Drawing for the job (mm, zero at the part's lowest x, y, z). A direction names the side the tool comes from. Round coordinates to 2 decimals unless told otherwise and drop trailing zeros. Write each loop counter-clockwise with the first axis right and the second up, starting at its lowest first coordinate (ties: lowest second). Pieces come first, ordered by that corner, then holes. Notation, with made-up numbers: (76, -28) - (108, -28) arc R18 cw to (108, -2) - close; hole circle Ø6 at (40.25, 53.25). An arc over 180 degrees is marked (long way). Answer in a Markdown table with one row per item.
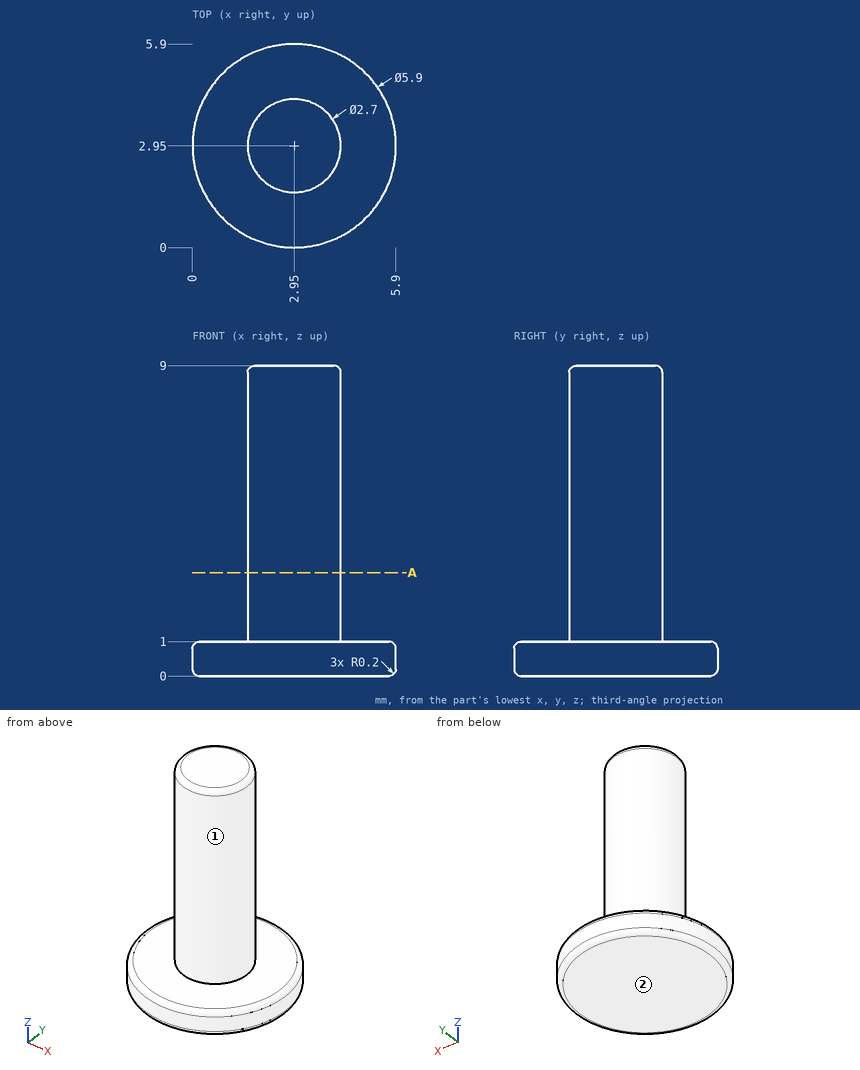
Q1. 3-axis set-ups, long thin cutter, end or side, ignore diameter. For the marked faces 1 and 2: which of +Z, -Z, +X, -X, +Y, -Y reach the whole face in a straight line?
Computed:
| item | result |
|---|---|
| face 1 | +Z |
| face 2 | -Z, +X, -X, +Y, -Y |
Q2. Drill centre lines: line 1 (Z direction, x = 4.6, y = 3.5); line 2 (Y direction, x = 2.1, z = 8.5); line 3 (X direction, y = 3.45, z = 8.25). Where is each one in solid material? Low to high.
Computed:
| item | result |
|---|---|
| line 1 | z = 0 to 1 |
| line 2 | y = 1.9 to 4 |
| line 3 | x = 1.7 to 4.2 |
Q3. Saw through at A-A on z = 3. List the corners of the cut face in (x, y).
Computed:
| item | result |
|---|---|
| outline | circle Ø2.7 at (2.95, 2.95) |
Q4. Flat gauge pins, fed straight in: pin 1 (3 mm diameter, centred on x = 2, y = 2, fed in from +Z); pin 2 (3 mm diameter, centred on y = 3, z = 3, fed in from +X). Where does each tip first touch, or does it go through?
Computed:
| item | result |
|---|---|
| pin 1 | stops at z = 9 |
| pin 2 | stops at x = 4.3 |
